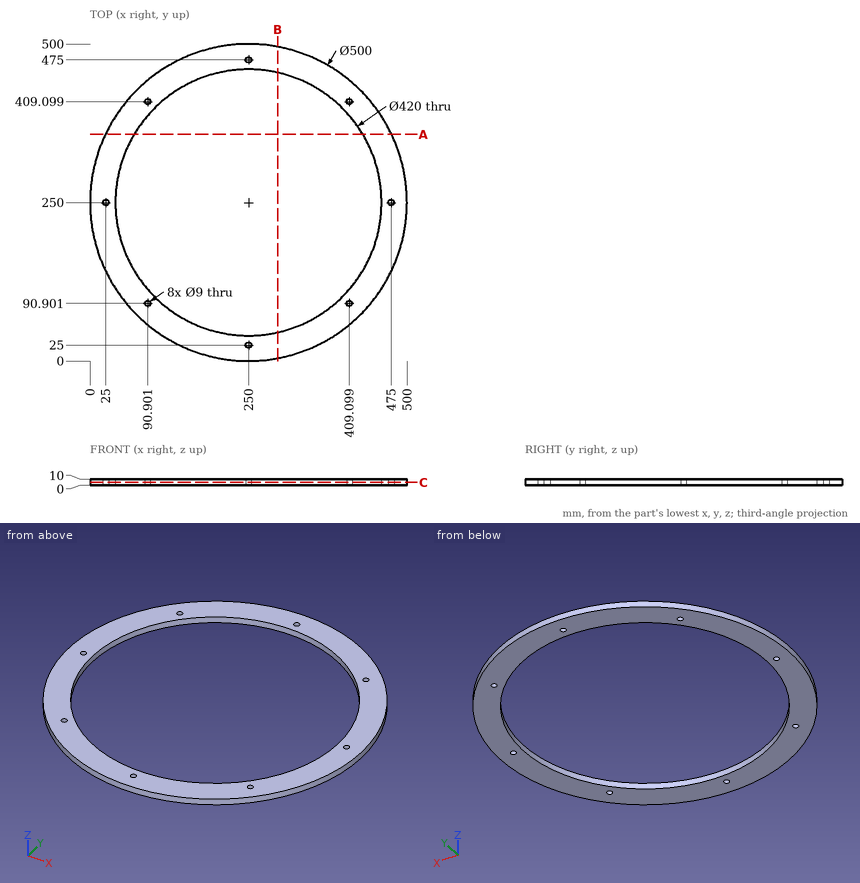
Can you work these out from the drawing? Everything is in mm from the part's minimum corner. Round coordinates to 2 decimals unless told otherwise and drop trailing zeros. Write each loop counter-clockwise with the first axis right and the second up, starting at its lowest first coordinate (ties: lowest second). Pieces come first, ordered by that corner, then holes.
1. Suppose I cut it at C-C (z = 4.5). State how many separate pieces and enclosed holes the cut face has, and give its area (3 significant figures).
2. I need wall thicknesses on L1, parallel to Y at x = 293.5, z = 8; L2, parallel to Y at x = 309.5, z = 9; L3, parallel to X at y = 416.5, z = 6. Which ranges of each line are inside material? Lowest first, please.
3. Suppose I cut it at B-B (x = 296). List the corners of the cut face in (y, z) for me.
4. Suppose I cut it at A-A (y = 357.5). List the corners of the cut face in (x, z) for me, and give its area (3 significant figures).
5. Will these pins go through, and if not, where does the flat tip stop? pin 1 Ø1.5 at (x, z) = (203, 1.5) entering from +Y; pin 2 Ø3 at (y, z) = (335, 1.5) entering from +X; pin 3 Ø1.5 at (y, z) = (414.5, 3) entering from -X.
Answer sheet:
1. separate pieces: 1
1. enclosed holes: 9
1. area: 57,300 mm2
2. L1: y = 3.81 to 44.55, 455.45 to 496.19
2. L2: y = 7.18 to 48.61, 451.39 to 492.82
2. L3: x = 63.51 to 122.02, 377.98 to 436.49
3. outline: (4.27, 0) - (45.1, 0) - (45.1, 10) - (4.27, 10) - close; (454.9, 0) - (495.73, 0) - (495.73, 10) - (454.9, 10) - close
4. outline: (24.29, 0) - (69.6, 0) - (69.6, 10) - (24.29, 10) - close; (430.4, 0) - (475.71, 0) - (475.71, 10) - (430.4, 10) - close
4. area: 906 mm2
5. pin 1: stops at y = 495.68
5. pin 2: stops at x = 485.64
5. pin 3: stops at x = 61.09
